Autodesk Inventor part; units mm, degrees
ref_plane "YZ Plane" through (0, 0, 0) normal (1, 0, 0) x (0, 1, 0)
ref_plane "XZ Plane" through (0, 0, 0) normal (0, 1, 0) x (-1, 0, 0)
ref_plane "XY Plane" through (0, 0, 0) normal (0, 0, 1) x (1, 0, 0)
sketch "Skizze1" plane through (0, 0, 0) normal (1, 0, 0) x (0, 1, 0)
  line L0 (4, 0) -> (4, 3)
  arc A0 (4, 3) -> (3, 4) centre (3, 3) ccw
  line L1 (3, 4) -> (0, 4)
  line L2 (0, 4) -> (0, 5)
  line L3 (0, 5) -> (-3, 5)
  line L4 (-3, 5) -> (-3, 2)
  line L5 (0, 0) -> (4, 0)
  line L6 (-3, 2) -> (-3, 0)
  line L7 (-3, 0) -> (0, 0)
  point P0 (0, 2)
  dimension "d0" = 2
  dimension "d1" = 4
  dimension "d2" = 3
  dimension "d3" = 5
  dimension "d4" = 3
  dimension "d5" = 1
  dimension "d6" = 1
revolve "Umdrehung1" add sketch "Skizze1" angle 360 about axis through (0, 0, 0) along (0, 1, 0)
sketch "Skizze2" plane through (0, 4, 0) normal (0, 1, 0) x (1, 0, 0)
  line L0 (-1.9622, -1.4344) -> (-1.9622, 1.4984) construction
  line L1 (-1.9622, 1.4984) -> (1.5378, 1.4984) construction
  line L2 (1.5378, 1.4984) -> (1.5378, -1.4344) construction
  line L3 (1.5378, -1.4344) -> (-1.9622, -1.4344) construction
  spline S0 degree 2 poles (0.4629, 1.2942) (0.7238, 1.2942) (1.1237, 1.0956) (1.2542, 0.9311) knots 0 0 0 1 2 2 2
  spline S1 degree 2 poles (1.2542, 0.9311) (1.4074, 0.7326) (1.5378, 0.2816) (1.5378, -0.0758) knots 0 0 0 1 2 2 2
  line L4 (1.5378, -0.0758) -> (1.5378, -1.0798)
  line L5 (1.5378, -1.0798) -> (-1.9622, -1.0798)
  line L6 (-1.9622, -1.0798) -> (-1.9622, -0.1523)
  spline S2 degree 2 poles (-1.9622, -0.1523) (-1.9622, 0.222) (-1.914, 0.5964) (-1.8204, 0.7666) knots 0 0 0 1 2 2 2
  spline S3 degree 2 poles (-1.8204, 0.7666) (-1.7211, 0.9566) (-1.3949, 1.1297) (-1.1737, 1.1297) knots 0 0 0 1 2 2 2
  spline S4 degree 2 poles (-1.1737, 1.1297) (-0.9269, 1.1297) (-0.5355, 0.8687) (-0.4249, 0.639) knots 0 0 0 1 2 2 2
  line L7 (-0.4249, 0.639) -> (-0.4079, 0.639)
  spline S5 degree 2 poles (-0.4079, 0.639) (-0.3228, 0.951) (0.1282, 1.2942) (0.4629, 1.2942) knots 0 0 0 1 2 2 2
  spline S6 degree 2 poles (0.4827, 0.8092) (0.2842, 0.8092) (0.0289, 0.6957) (-0.0618, 0.5255) knots 0 0 0 1 2 2 2
  spline S7 degree 2 poles (-0.0618, 0.5255) (-0.1186, 0.4149) (-0.1526, 0.154) (-0.1526, -0.0871) knots 0 0 0 1 2 2 2
  line L8 (-0.1526, -0.0871) -> (-0.1526, -0.6147)
  line L9 (-0.1526, -0.6147) -> (1.1407, -0.6147)
  line L10 (1.1407, -0.6147) -> (1.1407, -0.2374)
  spline S8 degree 2 poles (1.1407, -0.2374) (1.1407, 0.0689) (1.084, 0.4206) (0.9933, 0.5567) knots 0 0 0 1 2 2 2
  spline S9 degree 2 poles (0.9933, 0.5567) (0.8997, 0.6872) (0.6671, 0.8092) (0.4827, 0.8092) knots 0 0 0 1 2 2 2
  spline S10 degree 2 poles (-1.1084, 0.6447) (-1.2332, 0.6447) (-1.4204, 0.5596) (-1.4743, 0.466) knots 0 0 0 1 2 2 2
  spline S11 degree 2 poles (-1.4743, 0.466) (-1.5367, 0.3525) (-1.5651, 0.0774) (-1.5651, -0.1694) knots 0 0 0 1 2 2 2
  line L11 (-1.5651, -0.1694) -> (-1.5651, -0.6147)
  line L12 (-1.5651, -0.6147) -> (-0.5412, -0.6147)
  line L13 (-0.5412, -0.6147) -> (-0.5412, -0.0871)
  spline S12 degree 2 poles (-0.5412, -0.0871) (-0.5412, 0.1313) (-0.5866, 0.3383) (-0.6575, 0.449) knots 0 0 0 1 2 2 2
  spline S13 degree 2 poles (-0.6575, 0.449) (-0.7255, 0.5567) (-0.9439, 0.6447) (-1.1084, 0.6447) knots 0 0 0 1 2 2 2
  point P0 (0, 0)
extrude "Extrusion1" cut sketch "Skizze2" against normal blind 0.5
sketch "Skizze4" plane through (0, -3, 0) normal (0, -1, 0) x (1, 0, 0)
  line L0 (-4.889, 0.75) -> (-6.889, 0.75)
  line L1 (-6.889, 0.75) -> (-6.889, -0.75)
  line L2 (-6.889, -0.75) -> (-4.889, -0.75)
  line L3 (-4.889, -0.75) -> (-4.889, 0.75)
  point P0 (0, 0)
  dimension "d15" = 1.5
  dimension "d16" = 2
  dimension "d17" = 0.75
extrude "Extrusion3" add sketch "Skizze4" against normal blind 3
properties part number "ButtonB_neu"
Could you check a few things on this model? Use its own coordinates, in mm. A direction names the side the tool comes from. Coordinates: 2 decimals unless noted, no trailing zeros. Write each loop counter-clockwise with the first axis right and the second up, starting at its lowest first coordinate (ties: lowest second). Pieces come first, ordered by that corner, then holes. Notation, with made-up numbers: (18, -9) -> (25, -9) arc R10 ccw to (25, -3) -> close; hole circle Ø10 at (16.5, 9.25). An arc over 180 degrees is marked (long way). Write item = value, one per line. Start each with the question number.
(1) Which directions (+Z, -Z, +X, -X, +Y, -Y) give clear straight access to the entire face, cutting with the end or side of a thin tool? Please do faces 1 (the face through (-6, -2, 0.75)), 2 (the face through (0.5, 4, -0.1)), 3 (the face through (-6, -2, -0.75)).
(2) I want a section at B-B (y = 1). Please give me the cut outline in (x, z), plus the area to 3 significant figures.
(3) I want a section at D-D (z = -4.5). Please give me the cut outline in (x, y).
(4) I want a section at A-A (x = -5.5). Please give me the cut outline in (y, z).
(5) Will these pins go through, and if not, where does the flat tip stop? pin 1 (2 mm diameter, centred on x = -6, y = -2, fed in from -Z); pin 2 (1 mm diameter, centred on y = -0.5, z = -2.5, fed in from +X); pin 3 (3 mm diameter, centred on y = -1.5, z = 1, fed in from +X); pin 4 (2 mm diameter, centred on y = 1.5, z = 2.5, fed in from +X).
(6) I want a section at C-C (y = 3.75). Give the number of separate pieces and of enclosed holes in the cut face, plus the area to 3 significant figures.
(7) I need wall thicknesses on line 1 (Y direction, x = -0.5, z = -0.5); line 2 (X direction, y = 3.75, z = 0); line 3 (Y direction, x = -1.5, z = 4). Which ranges of each line are inside material? Lowest first, please. Write a range as [from, to].
(8) We'd pull the mould along X, two halves only. Please class faces 4 (the face through (0, 3.5, -1)), 5 (the face through (-6.889, -2, 0)), 6 (the face through (3.905, 1.479, -0.867)): released by +X, released by -X, zero draft, split by the parting line, or undercut.
Result set:
q1.face_1 = +Z, -X, +Y, -Y
q1.face_2 = +Z, -Z, +X, -X, +Y
q1.face_3 = -Z, -X, +Y, -Y
q2.outline = circle Ø8 at (0, 0)
q2.area = 50.3 mm2
q3.outline = (-2.18, -3) -> (2.18, -3) -> (2.18, 0) -> (-2.18, 0) -> close
q4.outline = (-3, -0.75) -> (0, -0.75) -> (0, 0.75) -> (-3, 0.75) -> close
q5.pin_1 = -0.75
q5.pin_2 = 4.58
q5.pin_3 = 5
q5.pin_4 = 3.71
q6.separate_pieces = 3
q6.enclosed_holes = 1
q6.area = 37.6 mm2
q7.line_1 = [-3, 3.5]
q7.line_2 = [-3.66, -1.96], [-1.56, -0.54], [-0.15, 1.14], [1.54, 3.66]
q7.line_3 = [-3, 0]
q8.face_4 = undercut
q8.face_5 = released by -X
q8.face_6 = split by the parting line
